Can you work these out from the model? Positions are in its coordinate system, mm. Face numbers are marked on the shaded views. Give positions to 0.01 mm unless a question says otherwise; leave off trailing zeros. Loops run counter-clockwise (first coordinate to the right, second up) from the corner with the lowest first, then second, coordinate; pieces in that order, holes last. Notation, with made-up numbers: (60.25, -38.75) - (115.25, -38.75) arc R10 ccw to (115.25, -20.75) - close; hole circle Ø1 at (88.25, 71.25). An arc over 180 degrees is marked (long way). Answer as a JSON object with one key per item and string values. Group by question number.
Item 1: Will these pins go through, and if not, where does the flat tip stop? pin 1 (1.5 mm diameter, centred on x = -2, z = 36, fed in from +Y); pin 2 (4 mm diameter, centred on x = -9, y = -27.5, fed in from +Z); pin 3 (1.5 mm diameter, centred on x = -9, z = 28.5, fed in from -Y).
Item 2: Thinking about a two-plate mould opening in Z: for the marked faces 1, 2 and 3, which applies, pulls with the +Z half, pulls with the -Z half, needs draft (parallel to the pull), parting line crosses it, or undercut?
Item 3: Suppose I cut it at B-B on x = -4. Write out the boundary of the cut face in (y, z), and give its area (3 significant figures).
Item 4: Please list where these lines run through material, in increasing order: L1, parallel to Z at x = -2.5, y = 0; L2, parallel to Y at x = 10.75, z = -1; L3, parallel to Z at x = -7.25, y = 0.
Item 5: Suppose I cut it at D-D on z = 0. Write out the boundary of the cut face in (x, y), and give its area (3 significant figures).
Item 6: Suppose I cut it at C-C on z = -31. Write out the boundary of the cut face in (x, y), and give its area (3 significant figures).
Item 7: Suppose I cut it at A-A on y = 0. Write out the boundary of the cut face in (x, z).
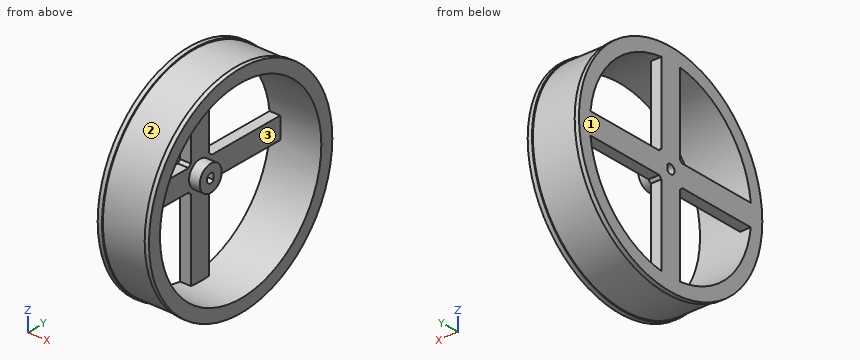
from build123d import *

# Parameters (mm, degrees)
SKETCH1_W               = 10
SKETCH1_H               = 6
SKETCH2_R               = 6
BOSS_EXTRUDE1_DEPTH     = 5
CUT_EXTRUDE1_DEPTH      = 15
CUT_EXTRUDE1_DEPTH_BACK = 11
CIRPATTERN1_COUNT       = 4


with BuildPart() as part:
    # Sketch1 → Revolve1 (revolve)
    with BuildSketch(Plane.XY):
        Polygon((-12, 50), (-12, 44), (12, 44), (12, 50), (10, 50), (10, 49.5), (-10, 49.5), (-10, 50), align=None)
        with Locations((-7, 3)):
            Rectangle(SKETCH1_W, SKETCH1_H)
    revolve(axis=Axis((0, 0, 0), (1, 0, 0)))

    # Sketch2 → Boss-Extrude1 (add)
    with BuildSketch(Plane(origin=(-12, 0, 0), x_dir=(0, 0, -1), z_dir=(1, 0, 0))):
        with BuildLine():
            Line((-5, 6.244997998), (-5, 43.714985989))
            ThreePointArc((-5, 43.714985989), (0, 44), (5, 43.714985989))
            Line((5, 43.714985989), (5, 6.244997998))
            ThreePointArc((5, 6.244997998), (0, -8), (-5, 6.244997998))
        make_face()
        Circle(SKETCH2_R, mode=Mode.SUBTRACT)
    boss_extrude1 = extrude(amount=BOSS_EXTRUDE1_DEPTH)

    # Sketch3 → Cut-Extrude1 (cut, two sides)
    with BuildSketch(Plane(origin=(-2, 0, 0), x_dir=(0, 0, -1), z_dir=(1, 0, 0))) as cut_extrude1_sk:
        with BuildLine():
            Line((-1.360147051, 1.6), (1.360147051, 1.6))
            ThreePointArc((1.360147051, 1.6), (0, -2.1), (-1.360147051, 1.6))
        make_face()
    extrude(amount=CUT_EXTRUDE1_DEPTH, mode=Mode.SUBTRACT)
    extrude(cut_extrude1_sk.sketch, amount=-CUT_EXTRUDE1_DEPTH_BACK, mode=Mode.SUBTRACT)

    # CirPattern1: Boss-Extrude1 ×4 about axis
    cirpattern1_axis = Axis((0, 0, 0), (1, 0, 0))
    for i in range(1, CIRPATTERN1_COUNT):
        add(boss_extrude1.rotate(cirpattern1_axis, i * 360 / CIRPATTERN1_COUNT))


solid = part.part
Worked out:
{
 "1": {"pin 1": "stops at y = 34.75", "pin 2": "stops at z = 42.85", "pin 3": "stops at y = -40.99"},
 "2": {"face 1": "needs draft", "face 2": "parting line crosses it", "face 3": "undercut"},
 "3": {"outline": "circle Ø99 at (0, 0); circle Ø12 at (0, 0); hole circle Ø88 at (0, 0); hole (1.6, -1.36) - (1.6, 1.36) arc R2.1 ccw (long way) to start", "area": "1,720 mm2"},
 "4": {"L1": "z = -49.5 to -44, -6 to -2.1, 2.1 to 6, 44 to 49.5", "L2": "y = -49.99 to -43.99, 43.99 to 49.99", "L3": "z = -49.5 to -2.1, 2.1 to 49.5"},
 "5": {"outline": "(-12, -50) - (-10, -50) - (-10, -49.5) - (10, -49.5) - (10, -50) - (12, -50) - (12, -44) - (-7, -44) - (-7, -6) - (-2, -6) - (-2, -2.1) - (-12, -2.1) - close; (-12, 1.6) - (-2, 1.6) - (-2, 6) - (-7, 6) - (-7, 44) - (12, 44) - (12, 50) - (10, 50) - (10, 49.5) - (-10, 49.5) - (-10, 50) - (-12, 50) - close", "area": "731 mm2"},
 "6": {"outline": "(-12, -39.23) - (-10, -39.23) - (-10, -38.59) - (10, -38.59) - (10, -39.23) - (12, -39.23) - (12, -31.22) - (-12, -31.22) - close; (-12, -5) - (-7, -5) - (-7, 5) - (-12, 5) - close; (-12, 31.22) - (12, 31.22) - (12, 39.23) - (10, 39.23) - (10, 38.59) - (-10, 38.59) - (-10, 39.23) - (-12, 39.23) - close", "area": "409 mm2"},
 "7": {"outline": "(-12, -50) - (-10, -50) - (-10, -49.5) - (10, -49.5) - (10, -50) - (12, -50) - (12, -44) - (-7, -44) - (-7, -6) - (-2, -6) - (-2, -2.1) - (-12, -2.1) - close; (-12, 2.1) - (-2, 2.1) - (-2, 6) - (-7, 6) - (-7, 44) - (12, 44) - (12, 50) - (10, 50) - (10, 49.5) - (-10, 49.5) - (-10, 50) - (-12, 50) - close"}
}
